Read the model definition and answer for the solid it produces. Units are mm, in the model's axes. Face numbers are marked on the shaded views. Coordinates: 2 decimals unless noted, no trailing zeros. Loops run counter-clockwise (first coordinate to the right, second up) from the corner with the lowest first, then second, coordinate; pieces in that order, holes last.
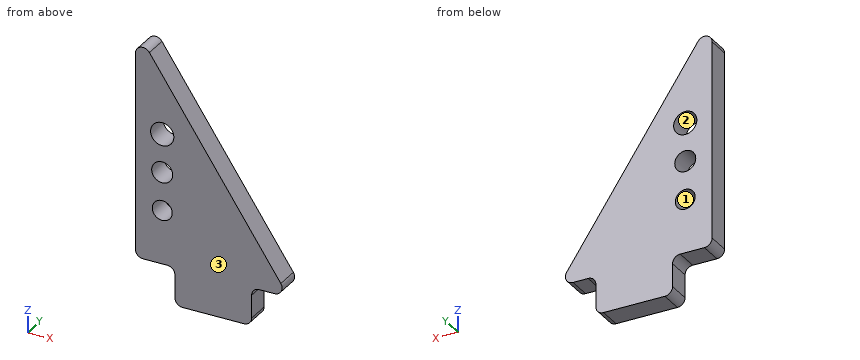
from build123d import *

# Parameters (mm, degrees)
SKETCH1_R           = 1.513481749
SKETCH1_R_2         = 1.371491644
SKETCH1_R_3         = 1.299503913
BOSS_EXTRUDE1_DEPTH = 3


with BuildPart() as part:
    # Sketch1 → Boss-Extrude1 (new body)
    with BuildSketch(Plane(origin=(0, 0, 0), x_dir=(1, 0, 0), z_dir=(0, 1, 0))):
        with BuildLine():
            Line((46.443482118, -40.25819894), (63.574965027, -14.560974577))
            ThreePointArc((63.574965027, -14.560974577), (63.624589331, -13.534416456), (62.742914732, -13.006274381))
            Line((62.742914732, -13.006274381), (60.767784216, -13.006274381))
            ThreePointArc((60.767784216, -13.006274381), (60.060677435, -12.713381162), (59.767784216, -12.006274381))
            Line((59.767784216, -12.006274381), (59.767784216, -9.006274381))
            ThreePointArc((59.767784216, -9.006274381), (59.474890998, -8.2991676), (58.767784216, -8.006274381))
            Line((58.767784216, -8.006274381), (50.767784216, -8.006274381))
            ThreePointArc((50.767784216, -8.006274381), (50.060677435, -8.2991676), (49.767784216, -9.006274381))
            Line((49.767784216, -9.006274381), (49.767784216, -12.006274381))
            ThreePointArc((49.767784216, -12.006274381), (49.474890998, -12.713381162), (48.767784216, -13.006274381))
            Line((48.767784216, -13.006274381), (45.611431824, -13.006274381))
            ThreePointArc((45.611431824, -13.006274381), (44.904325043, -13.2991676), (44.611431824, -14.006274381))
            Line((44.611431824, -14.006274381), (44.611431824, -39.703498743))
            ThreePointArc((44.611431824, -39.703498743), (45.321647675, -40.66059077), (46.443482118, -40.25819894))
        make_face()
        with Locations(Location((48.111431824, -30.006274381, 0), (0, 0, 270))):
            Circle(SKETCH1_R, mode=Mode.SUBTRACT)
        with Locations(Location((48.111431824, -25.006274381, 0), (0, 0, 270))):
            Circle(SKETCH1_R_2, mode=Mode.SUBTRACT)
        with Locations(Location((48.111431824, -20.006274381, 0), (0, 0, 270))):
            Circle(SKETCH1_R_3, mode=Mode.SUBTRACT)
    extrude(amount=BOSS_EXTRUDE1_DEPTH)


solid = part.part
Item 1: A cutting plane is placed at C-C on z = 20. Determine the outline of the cut face in (x, y), then the cut area to 3 significant figures.
Numbers:
outline: (44.61, 0) - (46.81, 0) - (46.81, 3) - (44.61, 3) - close; (49.41, 0) - (59.95, 0) - (59.95, 3) - (49.41, 3) - close
area: 38.2 mm2
Item 2: A cutting plane is placed at A-A on z = 29.5. Determine the outline of the cut face in (x, y).
Numbers:
outline: (44.61, 0) - (46.69, 0) - (46.69, 3) - (44.61, 3) - close; (49.54, 0) - (53.62, 0) - (53.62, 3) - (49.54, 3) - close
Item 3: Given pin 1 (0.9 mm diameter, centred on y = 1.5, z = 11, fed in from -X); pin 2 (1.8 mm diameter, centred on x = 48.11, z = 30.01, fed in from -Y); pin 3 (1.5 mm diameter, centred on y = 1, z = 10, fed in from +X), each flat-ended and moving along its own axis, determine where each tip first touches the part or whether it passes through.
Numbers:
pin 1: stops at x = 49.77
pin 2: passes through
pin 3: stops at x = 59.77
Item 4: A cutting plane is placed at B-B on y = 1.8. Determine the outline of the cut face in (x, z), then the cut area to 3 significant figures.
Numbers:
outline: (44.61, 14.01) arc R1 ccw to (45.61, 13.01) - (48.77, 13.01) arc R1 cw to (49.77, 12.01) - (49.77, 9.01) arc R1 ccw to (50.77, 8.01) - (58.77, 8.01) arc R1 ccw to (59.77, 9.01) - (59.77, 12.01) arc R1 cw to (60.77, 13.01) - (62.74, 13.01) arc R1 ccw to (63.57, 14.56) - (46.44, 40.26) arc R1 ccw to (44.61, 39.7) - close; hole circle Ø3.03 at (48.11, 30.01); hole circle Ø2.74 at (48.11, 25.01); hole circle Ø2.6 at (48.11, 20.01)
area: 329 mm2
Item 5: Determine the mould class of the marked faces 1, 2 and 3 for opening direction Z: released by +Z, released by -Z, zero draft, split by the parting line, or undercut.
Numbers:
face 1: undercut
face 2: undercut
face 3: zero draft
Item 6: A cutting plane is placed at D-D on x = 52.5. Determine the outline of the cut face in (y, z), then the cut area to 3 significant figures.
Numbers:
outline: (0, 8.01) - (3, 8.01) - (3, 31.17) - (0, 31.17) - close
area: 69.5 mm2
Item 7: Find the intervals of material crossed by line 1 along Z through (x, y) = (48.5, 2.1); line 2 along Z through (x, y) = (47.75, 0.55); line 3 along X through (y, z) = (2.65, 21), in increasing order.
Numbers:
line 1: z = 13.01 to 18.77, 21.25 to 23.69, 26.32 to 28.54, 31.47 to 37.17
line 2: z = 13.01 to 18.76, 21.25 to 23.68, 26.33 to 28.54, 31.48 to 38.3
line 3: x = 44.61 to 47.27, 48.95 to 59.28
